Check sheet for the modelled part. Datum: model origin and axes. Units: mm. Face numbers are marked on the shaded views. Give positions to 0.01 mm unless a question says otherwise; leave off trailing zeros. Order: outer loops, then holes, each group sorted by start corner. A loop starts at its lowest first (then second) coordinate and runs counter-clockwise, first axis right, second up.
Item 1: Material ranges on line 1 along X through (y, z) = (1.1, 12.75); line 2 along Y through (x, z) = (24.5, 10.5); line 3 along X through (y, z) = (3.7, 8), recorded low to high.
Item 2: Sectioned sample at B-B on y = 0.8. Record the boundary of the cut face in (x, z), and give its area (3 significant figures).
Item 3: Release check for a two-part mould opening along X. For the marked faces 1 and 2 record: released by +X, released by -X, zero draft, split by the parting line, or undercut.
Item 4: Gauge pin test, flat ends, axial feed: P1, Ø1, axis at y = 3.5, z = 0, coming from the +X side; P2, Ø1, axis at y = 3, z = 0, coming from the -X side; P3, Ø0.8, axis at y = 2.5, z = 15.5, coming from the -X side. Record the tip position at first contact, or that the pin passes through.
Item 5: Sectioned sample at C-C on x = 8. Record the boundary of the cut face in (y, z).
Item 6: Sectioned sample at D-D on z = 10. Record the boundary of the cut face in (x, y), and give its area (3 significant figures).
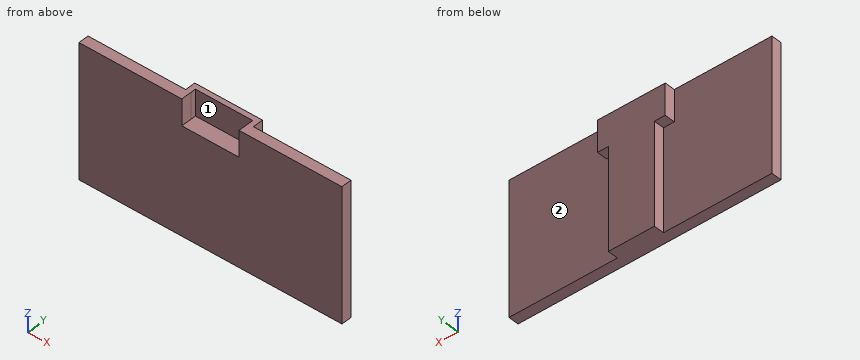
from build123d import *

# Parameters (mm, degrees)
SKETCH1_W                = 50.5
SKETCH1_H                = 25.5
BOSS_EXTRUDE1_DEPTH      = 2
SKETCH2_W                = 11
SKETCH2_H                = 5
CUT_EXTRUDE1_DEPTH       = 2
SKETCH3_W                = 8.85
SKETCH3_H                = 20.5
BOSS_EXTRUDE2_DEPTH      = 1
MOVE_FACE1_BY            = 1
SKETCH4_W                = 8.85
SKETCH4_H                = 1
BOSS_EXTRUDE3_DEPTH      = 5
BOSS_EXTRUDE4_DEPTH      = 2
BOSS_EXTRUDE4_DEPTH_BACK = 11
SKETCH5_W                = 5
SKETCH5_H                = 1
MOVE_FACE3_BY            = 0.15
MOVE_FACE4_BY            = 0.08
MOVE_FACE5_BY            = 0.08
SKETCH8_W                = 1
SKETCH8_H                = 5
BOSS_EXTRUDE5_DEPTH      = 1
SKETCH9_W                = 2.08
SKETCH9_H                = 1
BOSS_EXTRUDE6_DEPTH      = 2
SKETCH10_W               = 2.08
SKETCH10_H               = 1
BOSS_EXTRUDE7_DEPTH      = 2


with BuildPart() as part:
    # Sketch1 → Boss-Extrude1 (new body)
    with BuildSketch(Plane(origin=(0, 0, 0), x_dir=(1, 0, 0), z_dir=(0, 1, 0))):
        with Locations((6.667134831, -4.132373596)):
            Rectangle(SKETCH1_W, SKETCH1_H)
    extrude(amount=BOSS_EXTRUDE1_DEPTH)

    # Sketch2 → Cut-Extrude1 (cut)
    with BuildSketch(Plane(origin=(0, 2, 0), x_dir=(1, 0, 0), z_dir=(0, 1, 0))):
        with Locations((6.667134831, -14.382373596)):
            Rectangle(SKETCH2_W, SKETCH2_H)
    extrude(amount=-CUT_EXTRUDE1_DEPTH, mode=Mode.SUBTRACT)



with BuildPart() as body_2:
    # Sketch3 → Boss-Extrude2 (new body)
    with BuildSketch(Plane(origin=(0, 2, 0), x_dir=(1, 0, 0), z_dir=(0, 1, 0))):
        with Locations((6.667134831, -1.632373596)):
            Rectangle(SKETCH3_W, SKETCH3_H)
    extrude(amount=BOSS_EXTRUDE2_DEPTH)

    # Move Face1: a face moved outward by 1.0
    extrude(body_2.faces().sort_by_distance((6.667134831, 3, 1.632373596))[0], amount=MOVE_FACE1_BY, dir=(0, 1, 0))

    # Sketch4 → Boss-Extrude3 (add)
    with BuildSketch(Plane.XY.offset(11.882373596)):
        with Locations((6.667134831, 3.5)):
            Rectangle(SKETCH4_W, SKETCH4_H)
    extrude(amount=BOSS_EXTRUDE3_DEPTH)

    # Sketch5 → Boss-Extrude4 (add, two sides: drawn at the far end of the back side and taken through both)
    with BuildSketch(Plane.ZY.offset(-2.242134831).offset(-BOSS_EXTRUDE4_DEPTH_BACK)):
        with Locations((14.382373596, 3.5)):
            Rectangle(SKETCH5_W, SKETCH5_H)
    extrude(amount=BOSS_EXTRUDE4_DEPTH + BOSS_EXTRUDE4_DEPTH_BACK)

    # Move Face3: a face moved inward by 0.15
    extrude(body_2.faces().sort_by_distance((13.242134831, 3.5, 14.382373596))[0], amount=MOVE_FACE3_BY, dir=(-1, 0, 0), mode=Mode.SUBTRACT)

    # Move Face4: a face moved outward by 0.08
    extrude(body_2.faces().sort_by_distance((0.242134831, 3.5, 14.382373596))[0], amount=MOVE_FACE4_BY, dir=(-1, 0, 0))

    # Move Face5: a face moved outward by 0.08
    extrude(body_2.faces().sort_by_distance((13.092134831, 3.5, 14.382373596))[0], amount=MOVE_FACE5_BY, dir=(1, 0, 0))


with BuildPart() as part_1:
    add(part.part)

    add(body_2.part)  # Boss-Extrude5 merges body 2
    # Sketch8 → Boss-Extrude5 (add)
    with BuildSketch(Plane.XZ.offset(-3)):
        with Locations((0.662134831, 14.382373596)):
            Rectangle(SKETCH8_W, SKETCH8_H)
        with Locations((12.672134831, 14.382373596)):
            Rectangle(SKETCH8_W, SKETCH8_H)
    extrude(amount=BOSS_EXTRUDE5_DEPTH)

    # Sketch9 → Boss-Extrude6 (add)
    with BuildSketch(Plane(origin=(0, 2, 0), x_dir=(1, 0, 0), z_dir=(0, 1, 0))):
        with Locations((12.132134831, -11.382373596)):
            Rectangle(SKETCH9_W, SKETCH9_H)
    extrude(amount=BOSS_EXTRUDE6_DEPTH)

    # Sketch10 → Boss-Extrude7 (add)
    with BuildSketch(Plane(origin=(0, 2, 0), x_dir=(1, 0, 0), z_dir=(0, 1, 0))):
        with Locations((1.202134831, -11.382373596)):
            Rectangle(SKETCH10_W, SKETCH10_H)
    extrude(amount=BOSS_EXTRUDE7_DEPTH)


solid = part_1.part
Report:
1. line 1: x = -18.58 to 1.17, 12.17 to 31.92
1. line 2: y = 0 to 2
1. line 3: x = 2.24 to 11.09
2. outline: (-18.58, -8.62) - (31.92, -8.62) - (31.92, 16.88) - (12.17, 16.88) - (12.17, 11.88) - (1.17, 11.88) - (1.17, 16.88) - (-18.58, 16.88) - close
2. area: 1,230 mm2
3. face 1: undercut
3. face 2: zero draft
4. P1: stops at x = 11.09
4. P2: stops at x = 2.24
4. P3: stops at x = 0.16
5. outline: (0, -8.62) - (4, -8.62) - (4, 16.88) - (3, 16.88) - (3, 11.88) - (0, 11.88) - close
6. outline: (-18.58, 0) - (31.92, 0) - (31.92, 2) - (11.09, 2) - (11.09, 4) - (2.24, 4) - (2.24, 2) - (-18.58, 2) - close
6. area: 119 mm2
